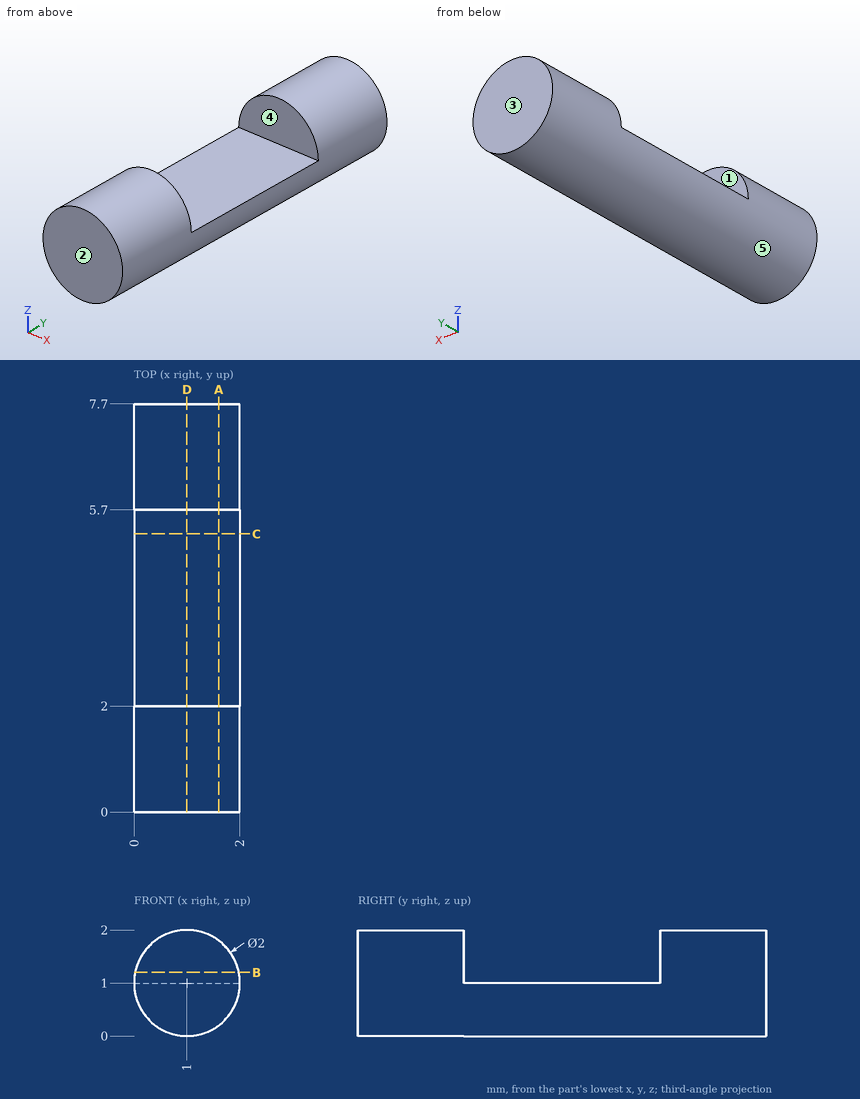
Here's the drawing with two shaded views (mm, measured from the low corner). I have some questions. A direction names the side the tool comes from. Round coordinates to 2 decimals unless told otherwise and drop trailing zeros. Loops run counter-clockwise (first coordinate to the right, second up) from the corner with the lowest first, then second, coordinate; pieces in that order, holes last. Notation, with made-up numbers: (49.5, 82.25) - (54.5, 82.25) arc R35 cw to (54.5, 114.25) - close; hole circle Ø4 at (78.25, 43.5). An arc over 180 degrees is marked (long way). Use CSV: the item, a comma, the result in double quotes. Start each with the question number.
1) For the marked faces 4 and 5, which set-ups out of +Z, -Z, +X, -X, +Y, -Y let a thin tool reach every point of the face, with its end or its side?
2) If we section it at A-A on x = 1.6: Write out the boundary of the cut face in (y, z), plus the area to 3 significant figures.
3) If we section it at C-C on y = 5.25: Write out the boundary of the cut face in (x, z).
4) If we section it at D-D on x = 1: Write out the boundary of the cut face in (y, z), plus the area to 3 significant figures.
5) We'd pull the mould along Y, two halves only. Please class the marked faces 1, 2 and 3: released by +Y, released by -Y, zero draft, split by the parting line, or undercut.
6) Please list where these lines run through material, in increasing order: probe 1 along Y at (x, z) = (1.4, 1.65); probe 2 along Z at (x, y) = (0.95, 6.75); probe 3 along Z at (x, y) = (0.6, 6). Write a range as [from, to].
7) If we section it at B-B on z = 1.2: Write out the boundary of the cut face in (x, y), plus the area to 3 significant figures.
Geometry results:
1,face 4,"+Z, +X, -X"
1,face 5,"+Y, -Y"
2,outline,"(0, 0.2) - (7.7, 0.2) - (7.7, 1.8) - (5.7, 1.8) - (5.7, 1) - (2, 1) - (2, 1.8) - (0, 1.8) - close"
2,area,"9.36 mm2"
3,outline,"(0, 1) arc R1 ccw to (2, 1) - close"
4,outline,"(0, 0) - (7.7, 0) - (7.7, 2) - (5.7, 2) - (5.7, 1) - (2, 1) - (2, 2) - (0, 2) - close"
4,area,"11.7 mm2"
5,face 1,"undercut"
5,face 2,"released by -Y"
5,face 3,"released by +Y"
6,probe 1,"y = [0, 2], [5.7, 7.7]"
6,probe 2,"z = [0, 2]"
6,probe 3,"z = [0.08, 1.92]"
7,outline,"(0.02, 0) - (1.98, 0) - (1.98, 2) - (0.02, 2) - close; (0.02, 5.7) - (1.98, 5.7) - (1.98, 7.7) - (0.02, 7.7) - close"
7,area,"7.84 mm2"
